Work out the finished part from the listing and answer in its coordinate system (mm). Give positions to 0.01 mm unless a question says otherwise; leave off trailing zeros. Write each loop counter-clockwise with the first axis right and the second up, starting at its lowest first coordinate (ties: lowest second). Pieces come first, ordered by that corner, then holes. Notation, with made-up numbers: (-12.75, 62) -> (-1.75, 62) arc R23 ccw to (-1.75, 73) -> close; hole circle Ø6 at (-24.75, 19.25). An arc over 180 degrees is marked (long way). Write item = value, one per line. Start each with the question number.
from build123d import *

# Parameters (mm, degrees)
SKETCH006_R   = 43
SKETCH006_R_2 = 1.5
SKETCH006_R_3 = 30
PAD_DEPTH     = 3


with BuildPart() as part:
    # Sketch006 → Pad (new body)
    with BuildSketch(Plane.XY.offset(22)):
        Circle(SKETCH006_R)
        with Locations((0, 36)):
            Circle(SKETCH006_R_2, mode=Mode.SUBTRACT)
        with Locations((31.176915, -18)):
            Circle(SKETCH006_R_2, mode=Mode.SUBTRACT)
        with Locations((-31.176915, -18)):
            Circle(SKETCH006_R_2, mode=Mode.SUBTRACT)
        Circle(SKETCH006_R_3, mode=Mode.SUBTRACT)
    extrude(amount=PAD_DEPTH)


solid = part.part
(1) A cutting plane is placed at C-C, the plane y = -18. Write down the section's boundary in (x, z).
(2) Determine the mould class of faces 1 (the cylindrical face through (-29.97, 1.32, 23.48)), 2 (the cylindrical face through (-5.598, 42.634, 23.479)), 3 (the flat face through (9, 29, 25)) for opening direction X: pulls with the +X half, pulls with the -X half, needs draft (parallel to the pull), parting line crosses it, or undercut.
(3) A cutting plane is placed at B-B, the plane z = 23.7. Write down the section's boundary in (x, y), then the cut area to 3 significant figures.
(4) A cutting plane is placed at A-A, the plane x = 0. Write down the section's boundary in (y, z), then the cut area to 3 significant figures.
(5) A cutting plane is placed at D-D, the plane y = -27.5. Write down the section's boundary in (x, z), then the cut area to 3 significant figures.
(6) Find the intervals of material crossed by line 1 along Y through (x, z) = (0, 22.9); line 2 along Y through (x, z) = (1, 23.45); line 3 along Y through (x, z) = (-17.5, 24.7), in increasing order.
(7) Each of these flat-tipped pins is pushed along its axis until it touches: pin 1 (5 mm diameter, centred on x = 0, y = 36, fed in from +Z); pin 2 (1.5 mm diameter, centred on y = -17.5, z = 22.5, fed in from -X). Where does it stop, or does it pass through?
Results list:
q1.outline = (-39.05, 22) -> (-32.68, 22) -> (-32.68, 25) -> (-39.05, 25) -> close; (-29.68, 22) -> (-24, 22) -> (-24, 25) -> (-29.68, 25) -> close; (24, 22) -> (29.68, 22) -> (29.68, 25) -> (24, 25) -> close; (32.68, 22) -> (39.05, 22) -> (39.05, 25) -> (32.68, 25) -> close
q2.face_1 = undercut
q2.face_2 = parting line crosses it
q2.face_3 = needs draft
q3.outline = circle Ø86 at (0, 0); hole circle Ø3 at (-31.18, -18); hole circle Ø60 at (0, 0); hole circle Ø3 at (0, 36); hole circle Ø3 at (31.18, -18)
q3.area = 2,960 mm²
q4.outline = (-43, 22) -> (-30, 22) -> (-30, 25) -> (-43, 25) -> close; (30, 22) -> (34.5, 22) -> (34.5, 25) -> (30, 25) -> close; (37.5, 22) -> (43, 22) -> (43, 25) -> (37.5, 25) -> close
q4.area = 69.0 mm²
q5.outline = (-33.06, 22) -> (-11.99, 22) -> (-11.99, 25) -> (-33.06, 25) -> close; (11.99, 22) -> (33.06, 22) -> (33.06, 25) -> (11.99, 25) -> close
q5.area = 126 mm²
q6.line_1 = -43 to -30, 30 to 34.5, 37.5 to 43
q6.line_2 = -42.99 to -29.98, 29.98 to 34.88, 37.12 to 42.99
q6.line_3 = -39.28 to -24.37, 24.37 to 39.28
q7.pin_1 = 25
q7.pin_2 = -39.6
